from build123d import *

# Parameters (mm, degrees)
BOSS_EXTRUDE1_DEPTH      = 314
BOSS_EXTRUDE1_DEPTH_BACK = 26
SKETCH1_R                = 8
SKETCH1_3_R              = 8
BOSS_EXTRUDE2_DEPTH      = 9
FILLET1_R                = 2
CHAMFER2_SIZE            = 2
CHAMFER3_SIZE            = 1.5
SKETCH2_OUTSIDE_W        = 129.284
SKETCH2_OUTSIDE_H        = 125.572
SKETCH2_OUTSIDE_R        = 12
CUT_EXTRUDE1_DEPTH       = 9
CUT_EXTRUDE1_DRAFT       = -60


with BuildPart() as part:
    # Sketch1 → Boss-Extrude1 (new, two sides: drawn at the far end of the back side and taken through both)
    with BuildSketch(Plane(origin=(0, 0, 0), x_dir=(1, 0, 0), z_dir=(0, 1, 0)).offset(-BOSS_EXTRUDE1_DEPTH_BACK)):
        with Locations(Location((0, 0, 0), (0, 0, 270))):
            Circle(SKETCH1_R)
    extrude(amount=BOSS_EXTRUDE1_DEPTH + BOSS_EXTRUDE1_DEPTH_BACK)

    # Sketch1_3 → Boss-Extrude2 (add)
    with BuildSketch(Plane(origin=(0, 0, 0), x_dir=(1, 0, 0), z_dir=(0, 1, 0))):
        Polygon((13.856406461, 0), (6.92820323, 12), (-6.92820323, 12), (-13.856406461, 0), (-6.92820323, -12), (6.92820323, -12), align=None)
        with Locations(Location((0, 0, 0), (0, 0, 270))):
            Circle(SKETCH1_3_R, mode=Mode.SUBTRACT)
    extrude(amount=BOSS_EXTRUDE2_DEPTH)

    # Fillet1
    fillet1_edges = [part.edges().sort_by_distance(p)[0] for p in [
        (0, 0, -8),
        (0, 9, -8),
    ]]
    fillet(fillet1_edges, radius=FILLET1_R)

    # Chamfer2
    chamfer2_edges = [part.edges().sort_by_distance(p)[0] for p in [
        (0, -26, -8),
    ]]
    chamfer(chamfer2_edges, length=CHAMFER2_SIZE)

    # Chamfer3
    chamfer3_edges = [part.edges().sort_by_distance(p)[0] for p in [
        (0, 314, -8),
    ]]
    chamfer(chamfer3_edges, length=CHAMFER3_SIZE)


with BuildPart() as cut_extrude1_tool:
    # Sketch2 outside → Cut-Extrude1 (with draft: the straight prism first)
    with BuildSketch(Plane(origin=(0, 9, 0), x_dir=(1, 0, 0), z_dir=(0, 1, 0))):
        Rectangle(SKETCH2_OUTSIDE_W, SKETCH2_OUTSIDE_H)
        Circle(SKETCH2_OUTSIDE_R, mode=Mode.SUBTRACT)
    extrude(amount=-CUT_EXTRUDE1_DEPTH)
    # Cut-Extrude1: the draft: its side faces are tilted about the plane it starts from
    cut_extrude1_sides = [cut_extrude1_tool.faces().sort_by_distance(p)[0] for p in [
        (0, 4.5, 62.786),
        (64.642, 4.5, 0),
        (0, 4.5, -62.786),
        (-64.642, 4.5, 0),
        (-12, 4.5, 0),
    ]]
    draft(cut_extrude1_sides, Plane(origin=(0, 9, 0), x_dir=(1, 0, 0), z_dir=(0, 1, 0)), CUT_EXTRUDE1_DRAFT)


with BuildPart() as part_1:
    add(part.part)

    # Cut-Extrude1: cut by cut_extrude1_tool
    add(cut_extrude1_tool.part, mode=Mode.SUBTRACT)


solid = part_1.part
Work out the finished part from the listing and answer in its coordinate system (mm). A direction names the side the tool comes from. Round coordinates to 2 decimals unless told otherwise and drop trailing zeros. Order: outer loops, then holes, each group sorted by start corner. A loop starts at its lowest first (then second) coordinate and runs counter-clockwise, first axis right, second up. Notation, with made-up numbers: M 51,26.5 L 77,26.5 A8 ccw 77,30.5 Z; hole C 88,-17 d10. An arc over 180 degrees is marked long. Put each result on its own line as item: value. Start each with the question number.
Q1. A tool of negligible diameter and unlimited length cuts with its end or side. For faces 1 (the flat face through (-5, 9, -9)), 2 (the flat face through (0, 314, 0)), 3 (the flat face through (3, 0, -10)), from which of +Z, -Z, +X, -X, +Y, -Y can it reach the whole face along a straight path? Write none if from no direction.
Q2. Straight lines are drawn through the part: L1, parallel to Y at x = -9.5, z = 4.25; L2, parallel to X at y = 140.5, z = -1. For each, find the intervals that lie inside material, in ascending order. Write a range as [from, to].
Q3. Section A-A, the plane y = 128 is taken. Write down the section's boundary in (x, z).
Q4. Flat-ended cylindrical pins translate along their axes: pin 1 (12 mm diameter, centred on x = -1.5, y = 267.5, fed in from -Z); pin 2 (6 mm diameter, centred on y = 227, z = -3, fed in from -X); pin 3 (3 mm diameter, centred on y = 134.5, z = 8.5, fed in from +X). Find the tip coordinate at first contact, or state that the pin passes through.
Findings below:
1. face 1: +Y
1. face 2: +Z, -Z, +X, -X, +Y
1. face 3: -Y
2. L1: y = [0, 9]
2. L2: x = [-7.94, 7.94]
3. outline: C 0,0 d16
4. pin 1: stops at z = -8
4. pin 2: stops at x = -8
4. pin 3: stops at x = 3.87
